```python
from build123d import *

# Parameters (mm, degrees)
SKETCH_1_R               = 3.8
SKETCH_1_R_2             = 2.6
EXTRUDE_1_DEPTH          = 17
CUT_EXTRUDE_1_DEPTH      = 17
PATTERN_CIRCULAR_1_COUNT = 2
PATTERN_CIRCULAR_1_ANGLE = 120
FILLET_1_R               = 2


with BuildPart() as part:
    # 스케치1 → 보스-돌출1 (new body)
    with BuildSketch(Plane.XY):
        Circle(SKETCH_1_R)
        Circle(SKETCH_1_R_2, mode=Mode.SUBTRACT)
    extrude(amount=EXTRUDE_1_DEPTH)

    # 스케치2 → 컷-돌출1 (cut)
    with BuildSketch(Plane(origin=(0, 0, 0), x_dir=(1, 0, 0), z_dir=(0, 1, 0))):
        with BuildLine():
            Line((-2, -8), (-2, -12))
            ThreePointArc((-2, -12), (0, -14), (2, -12))
            Line((2, -12), (2, -8))
            ThreePointArc((2, -8), (0, -6), (-2, -8))
        make_face()
    cut_extrude_1 = extrude(amount=-CUT_EXTRUDE_1_DEPTH, mode=Mode.SUBTRACT)

    # 원형 패턴1: 컷-돌출1 ×2 about axis
    pattern_circular_1_axis = Axis((0, 0, 0), (0, 0, 1))
    for i in range(1, PATTERN_CIRCULAR_1_COUNT):
        add(cut_extrude_1.rotate(pattern_circular_1_axis, i * PATTERN_CIRCULAR_1_ANGLE / (PATTERN_CIRCULAR_1_COUNT - 1)), mode=Mode.SUBTRACT)

    # 필렛1
    # the kernel refuses this fillet: 2 mm, written as the material it takes off along each edge
    with BuildSketch(Plane(origin=(0, 0, 0), x_dir=(1, 0, 0), z_dir=(0, -1, 0))) as fillet_1_piece_1:
        with BuildLine():
            CenterArc((1.8, 1.833030278), FILLET_1_R, 293.578178478, 66.421821522)
            Line((2.6, 0), (2.616, -0.036660606))
            ThreePointArc((2.616, -0.036660606), (3.2, -0.04), (3.8, -0.04))
            Line((3.8, -0.04), (3.84, 0))
            Line((3.84, 0), (3.84, 1.833030278))
            Line((3.84, 1.833030278), (3.8, 1.833030278))
        make_face()
    revolve(axis=Axis((0, 0, 0), (0, 0, 1)), mode=Mode.SUBTRACT)


solid = part.part
```
Input: part model. Units: mm. Frame: model coordinates. A direction names the side the tool comes from. Give positions to 0.01 mm unless a question says otherwise; leave off trailing zeros. Order: outer loops, then holes, each group sorted by start corner. A loop starts at its lowest first (then second) coordinate and runs counter-clockwise, first axis right, second up.
1. Cut plane B-B (x = 0). State how many separate pieces and enclosed holes the cut face has, and give its area (3 significant figures).
Computed:
separate pieces: 3
enclosed holes: 0
area: 30.0 mm2
2. Cut plane A-A (z = 9). Return loops of the section in (x, y), and give its area (3 significant figures).
Computed:
outline: (-2, -3.23) - (-2, -1.66) arc R2.6 cw to (0.44, 2.56) - (1.8, 3.35) arc R3.8 ccw to start; (2, -3.23) arc R3.8 ccw to (3.8, -0.12) - (2.44, -0.9) arc R2.6 cw to (2, -1.66) - close
area: 13.7 mm2
3. Draft query along X for faces 1 (the face through (-2.8, 2.57, 9.31)), 2 (the face through (1.11, 2.95, 10.03)), 3 (the face through (3.109, -0.514, 9.972)), 4 (the face through (2, -2, 17)). Return one class per face: released by +X, released by -X, zero draft, split by the parting line, or undercut.
Computed:
face 1: split by the parting line
face 2: released by +X
face 3: undercut
face 4: zero draft
4. Cut plane C-C (z = 4). Return loops of the section in (x, y).
Computed:
outline: circle Ø7.6 at (0, 0); hole circle Ø5.2 at (0, 0)
5. Pin query (flat end, axial travel): pin 1 Ø2 at (y, z) = (2, 2.5) entering from -X; pin 2 Ø1.7 at (y, z) = (-2, 10.5) entering from -X; pin 3 Ø1 at (x, z) = (-3, 8.5) entering from -Y. Return the tip coordinate at first contact, or that it passes through.
Computed:
pin 1: stops at x = -3.67
pin 2: stops at x = -3.62
pin 3: stops at y = -2.86
6. Line query: probe 1 along Y at (x, z) = (0, 3.75); probe 2 along X at (y, z) = (-1.5, 12.5); probe 3 along X at (y, z) = (-1.25, 5.5). Output: solid intervals per line, ascending.
Computed:
probe 1: y = -3.8 to -2.6, 2.6 to 3.8
probe 2: x = -3.49 to -2.12, 2.12 to 3.49
probe 3: x = -3.59 to -2.28, 2.28 to 3.59
7. Set-up query: faces 5 (the face through (-1.916, 1.757, 8.381)), 6 (the face through (0, -3, 6)), 7 (the face through (2, -2, 10)), 8 (the face through (2.6, 1.4, 14)). Return all of +Z, -Z, +X, -X, +Y, -Y with unobstructed straight access to the full face (end or side cutting, diameter ignored); none if empty.
Computed:
face 5: +Z, -Z
face 6: -Y
face 7: +Y, -Y
face 8: none
